from build123d import *

# Parameters (mm, degrees)
PAD021_DEPTH                        = 3
SKETCH083_R                         = 1.7
POCKET041_DEPTH                     = 0.001
POCKET041_DEPTH_BACK                = 3.001
SKETCH084_R                         = 1.7
POCKET042_DEPTH                     = 0.001
POCKET042_DEPTH_BACK                = 3.001
BODY001003005003013_PLACEMENT_ANGLE = 60
CLONE020_PLACEMENT_ANGLE            = 60


with BuildPart() as part:
    # Sketch082 → Pad021 (new body)
    with BuildSketch(Plane.XY):
        with BuildLine():
            ThreePointArc((156.627412, 120.879551), (87.258751, 177.56667), (0, 197.848457))
            Line((0, 197.848457), (0, 182.848457))
            ThreePointArc((144.752611, 111.714995), (80.643177, 164.104346), (0, 182.848457))
            ThreePointArc((148.102078, 107.234942), (146.444477, 109.487778), (144.752611, 111.714995))
            ThreePointArc((148.102078, 107.234942), (148.703343, 106.843433), (149.41205, 106.955386))
            Line((155.154429, 110.27075), (149.41205, 106.955386))
            Line((155.154429, 110.27075), (160.726477, 113.487773))
            ThreePointArc((160.726477, 113.487773), (161.203737, 114.141753), (161.040435, 114.934722))
            ThreePointArc((161.040435, 114.934722), (158.861734, 117.927781), (156.627412, 120.879551))
        make_face()
    pad021 = extrude(amount=PAD021_DEPTH)

    # Mirrored029: Pad021 across Sketch082 V_Axis
    add(pad021.mirror(Plane(origin=(0, 0, 0), x_dir=(0, 0, 1), z_dir=(1, 0, 0))))

    # Sketch083 → Pocket041 (cut, two sides)
    with BuildSketch(Plane.XY) as pocket041_sk:
        with Locations((149.149219, 118.266841)):
            Circle(SKETCH083_R)
        with Locations((-149.149219, 118.266841)):
            Circle(SKETCH083_R)
    extrude(amount=-POCKET041_DEPTH, mode=Mode.SUBTRACT)
    extrude(pocket041_sk.sketch, amount=POCKET041_DEPTH_BACK, mode=Mode.SUBTRACT)

    # Sketch084 → Pocket042 (cut, two sides)
    with BuildSketch(Plane.XY) as pocket042_sk:
        with Locations((0, 190.348457)):
            Circle(SKETCH084_R)
    extrude(amount=-POCKET042_DEPTH, mode=Mode.SUBTRACT)
    extrude(pocket042_sk.sketch, amount=POCKET042_DEPTH_BACK, mode=Mode.SUBTRACT)


with BuildPart() as part_1:
    # Body001003005003013 placement: moved
    add(part.part.rotate(Axis((0, 0, 0), (0, 0, 1)), BODY001003005003013_PLACEMENT_ANGLE))


with BuildPart() as part_2:
    # Clone020 placement: moved
    add(part_1.part.moved(Location((1314, 822, 0))).rotate(Axis((1314, 822, 0), (0, 0, -1)), CLONE020_PLACEMENT_ANGLE))


solid = part_2.part
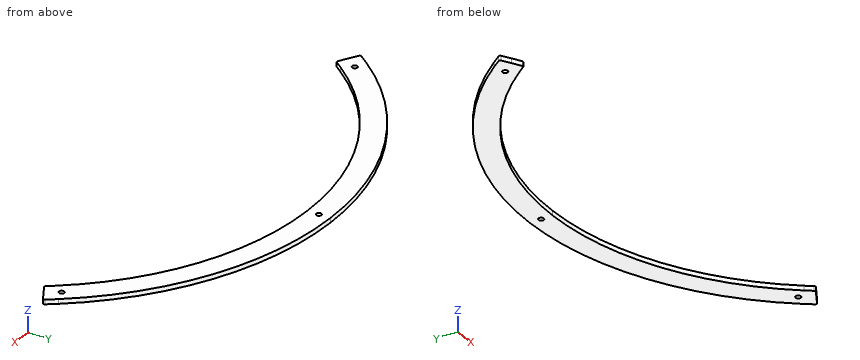
The model under review builds one solid part; all positions refer to its coordinate system, in mm. Round coordinates to 2 decimals unless told otherwise and drop trailing zeros. Loops run counter-clockwise (first coordinate to the right, second up) from the corner with the lowest first, then second, coordinate; pieces in that order, holes last. Notation, with made-up numbers: (-13.5, -14.75) -> (41.5, -14.75) arc R25 cw to (41.5, 21.25) -> close; hole circle Ø9 at (-22, 8). An arc over 180 degrees is marked (long way). Write item = value, one per line. Start each with the question number.
Item 1: To check wall thickness, follow L1, parallel to X at y = 935.5, z = 1.55; L2, parallel to X at y = 938, z = 0.65; L3, parallel to Y at x = 1313, z = 0.8. State the ranges of each line that lie inside material, in increasing order.
Item 2: Insertion check: pin 1 (1 mm diameter, centred on x = 1231, z = 1, fed in from +Y); pin 2 (1 mm diameter, centred on y = 961, z = 2, fed in from -X); pin 3 (1.5 mm diameter, centred on x = 1440.5, z = 2.5, fed in from -Y) (3 decimals). Each pin has a flat end and moves straight along its axis. Give the tip position at first contact, or say it passes through.
Item 3: Take a section at C-C on y = 968.5. Give the boundary of the cut face in (x, z), plus the area to 3 significant figures.
Item 4: Take a section at D-D on x = 1395.5. Give the boundary of the cut face in (y, z), plus the area to 3 significant figures.
Item 5: Take a section at B-B on z = 2.2. Give the boundary of the cut face in (x, y) (3 decimals).
Item 6: Take a section at A-A on y = 982.5. Give the boundary of the cut face in (x, z).
Result:
q1.L1 = 1153.25 to 1170.64, 1457.36 to 1474.75
q1.L2 = 1153.73 to 1172.66, 1455.34 to 1474.27
q1.L3 = 1004.85 to 1010.97, 1013.72 to 1019.85
q2.pin_1 = 1001.83
q2.pin_2 = 1172.71
q2.pin_3 = 953.305
q3.outline = (1181.03, 0) -> (1204.59, 0) -> (1204.59, 3) -> (1181.03, 3) -> close; (1423.41, 0) -> (1446.97, 0) -> (1446.97, 3) -> (1423.41, 3) -> close
q3.area = 141 mm²
q4.outline = (985.68, 0) -> (1002.28, 0) -> (1002.28, 3) -> (985.68, 3) -> close
q4.area = 49.8 mm²
q5.outline = (1152.96, 936.935) arc R1 ccw to (1153.274, 935.488) -> (1164.588, 928.955) arc R1 ccw to (1165.898, 929.235) arc R182.849 cw to (1169.247, 933.715) arc R182.848 cw to (1314, 1004.848) arc R182.848 cw to (1458.753, 933.715) arc R182.849 cw to (1462.102, 929.235) arc R1 ccw to (1463.412, 928.955) -> (1474.726, 935.488) arc R1 ccw to (1475.04, 936.935) arc R197.848 ccw to (1470.627, 942.88) arc R197.848 ccw to (1157.373, 942.88) arc R197.848 ccw to start; hole circle Ø3.4 at (1164.851, 940.267); hole circle Ø3.4 at (1314, 1012.348); hole circle Ø3.4 at (1463.149, 940.267)
q6.outline = (1198.31, 0) -> (1226.4, 0) -> (1226.4, 3) -> (1198.31, 3) -> close; (1401.6, 0) -> (1429.69, 0) -> (1429.69, 3) -> (1401.6, 3) -> close
